The model under review builds one solid part; all positions refer to its coordinate system, in mm. Face numbers are marked on the shaded views. Round coordinates to 2 decimals unless told otherwise and drop trailing zeros. Order: outer loops, then holes, each group sorted by start corner. A loop starts at its lowest first (then second) coordinate and runs counter-clockwise, first axis right, second up. Notation, with made-up numbers: (8.25, 5) -> (36.25, 5) arc R17 ccw to (36.25, 31) -> close; hole circle Ø3 at (39, 27). An arc over 180 degrees is marked (long way). Use a Markdown table: item, result. Add a question column.
```python
from build123d import *

# Parameters (mm, degrees)
F0_R     = 11.1
F1_DEPTH = 7
F2_R     = 7.5
F3_SIZE  = 2.3333333333


with BuildPart() as f1:
    # F0 (on Top) → F1 (new body)
    with BuildSketch(Plane.XY):
        with BuildLine():
            ThreePointArc((13.75, -8.3754104377), (15.5013709071, -4.3494252494), (16.1, 0))
            ThreePointArc((16.1, 0), (15.5013709071, 4.3494252494), (13.75, 8.3754104377))
            ThreePointArc((13.75, 8.3754104377), (11.4, 0), (13.75, -8.3754104377))
        make_face()
        with BuildLine():
            ThreePointArc((13.75, 8.3754104377), (15.5013709071, 4.3494252494), (16.1, 0))
            ThreePointArc((16.1, 0), (15.5013709071, -4.3494252494), (13.75, -8.3754104377))
            ThreePointArc((13.75, -8.3754104377), (31.8494252494, -15.5013709071), (43.6, 0))
            ThreePointArc((43.6, 0), (31.8494252494, 15.5013709071), (13.75, 8.3754104377))
        make_face()
        with Locations((27.5, 0)):
            Circle(F0_R, mode=Mode.SUBTRACT)
        with BuildLine():
            ThreePointArc((13.75, -8.3754104377), (11.4, 0), (13.75, 8.3754104377))
            ThreePointArc((13.75, 8.3754104377), (0, 16.1), (-13.75, 8.3754104377))
            ThreePointArc((-13.75, 8.3754104377), (-11.9986290929, 4.3494252494), (-11.4, 0))
            ThreePointArc((-11.4, 0), (-11.9986290929, -4.3494252494), (-13.75, -8.3754104377))
            ThreePointArc((-13.75, -8.3754104377), (0, -16.1), (13.75, -8.3754104377))
        make_face()
        Circle(F0_R, mode=Mode.SUBTRACT)
        with BuildLine():
            ThreePointArc((-11.4, 0), (-11.9986290929, 4.3494252494), (-13.75, 8.3754104377))
            ThreePointArc((-13.75, 8.3754104377), (-16.1, 0), (-13.75, -8.3754104377))
            ThreePointArc((-13.75, -8.3754104377), (-11.9986290929, -4.3494252494), (-11.4, 0))
        make_face()
        with BuildLine():
            ThreePointArc((-13.75, -8.3754104377), (-16.1, 0), (-13.75, 8.3754104377))
            ThreePointArc((-13.75, 8.3754104377), (-43.6, 0), (-13.75, -8.3754104377))
        make_face()
        with Locations((-27.5, 0)):
            Circle(F0_R, mode=Mode.SUBTRACT)
    extrude(amount=F1_DEPTH)

    # F2
    f2_edges = [f1.edges().sort_by_distance(p)[0] for p in [
        (-13.75, 8.37541, 3.5),
        (13.75, 8.37541, 3.5),
        (-13.75, -8.37541, 3.5),
        (13.75, -8.37541, 3.5),
    ]]
    fillet(f2_edges, radius=F2_R)

    # F3
    f3_edges = [f1.edges().sort_by_distance(p)[0] for p in [
        (0, 16.1, 7),
        (-13.75, 11.680654, 7),
        (-43.6, 0, 0),
    ]]
    chamfer(f3_edges, length=F3_SIZE)


solid = f1.part
```
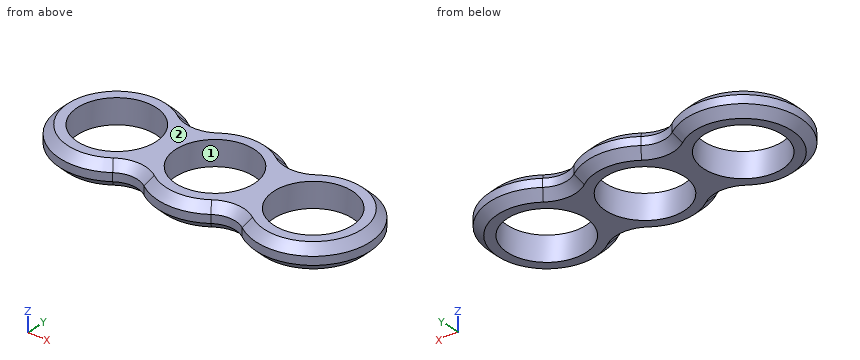
Q1. For pin 1 (3 mm diameter, centred on y = -5, z = 5, fed in from -X); pin 2 (18 mm diameter, centred on x = -27.5, y = 0, fed in from +Z); pin 3 (1.5 mm diameter, centred on x = -32, z = 2, fed in from +Y); pin 4 (1 mm diameter, centred on y = 0.5, z = 5.5, fed in from +X), all flat-tipped, find the tip position at first contact; note any pin that passes through.
Q2. To check wall thickness, follow line 1 along X through (y, z) = (2, 1.75); line 2 along X through (y, z) = (-1.5, 3.25); line 3 along Y through (x, z) = (-27.5, 3.75). State the ranges of each line that lie inside material, in increasing order.
Q3. Add section C-C, the plane z = 1.5. Give the number of separate pieces and of enclosed holes in the cut face, then the cut area to 3 significant figures.
Q4. Add section B-B, the plane y = 0. Give the boundary of the cut face in (x, z), then the cut area to 3 significant figures.
Q5. Draft analysis for pull direction X (two halves, no side actions). For the marked faces 1 and 2, state which applies: released by +X, released by -X, zero draft, split by the parting line, or undercut.
Q6. Add section A-A, the plane x = -27.5. Give the boundary of the cut face in (y, z), then the cut area to 3 significant figures.
Return value:
| question | item | result |
|---|---|---|
| 1 | pin 1 | x = -43.21 |
| 1 | pin 2 | through |
| 1 | pin 3 | y = 15.64 |
| 1 | pin 4 | x = 43.26 |
| 2 | line 1 | -42.89 to -38.42, -16.58 to -10.92, 10.92 to 16.58, 38.42 to 42.89 |
| 2 | line 2 | -43.53 to -38.5, -16.5 to -11, 11 to 16.5, 38.5 to 43.53 |
| 2 | line 3 | -16.1 to -11.1, 11.1 to 16.1 |
| 3 | separate pieces | 1 |
| 3 | enclosed holes | 3 |
| 3 | area | 1,030 mm² |
| 4 | outline | (-43.6, 2.33) -> (-41.27, 0) -> (-38.6, 0) -> (-38.6, 7) -> (-41.27, 7) -> (-43.6, 4.67) -> close; (-16.4, 0) -> (-11.1, 0) -> (-11.1, 7) -> (-16.4, 7) -> close; (11.1, 0) -> (16.4, 0) -> (16.4, 7) -> (11.1, 7) -> close; (38.6, 0) -> (41.27, 0) -> (43.6, 2.33) -> (43.6, 4.67) -> (41.27, 7) -> (38.6, 7) -> close |
| 4 | area | 133 mm² |
| 5 | face 1 | undercut |
| 5 | face 2 | zero draft |
| 6 | outline | (-16.1, 2.33) -> (-13.77, 0) -> (-11.1, 0) -> (-11.1, 7) -> (-13.77, 7) -> (-16.1, 4.67) -> close; (11.1, 0) -> (13.77, 0) -> (16.1, 2.33) -> (16.1, 4.67) -> (13.77, 7) -> (11.1, 7) -> close |
| 6 | area | 59.1 mm² |
